Autodesk Inventor part; units mm, degrees
ref_plane "YZ Plane" through (0, 0, 0) normal (1, 0, 0) x (0, 1, 0)
ref_plane "XZ Plane" through (0, 0, 0) normal (0, 1, 0) x (-1, 0, 0)
ref_plane "XY Plane" through (0, 0, 0) normal (0, 0, 1) x (1, 0, 0)
sketch "Sketch1" plane through (0, 0, 0) normal (0, 1, 0) x (-1, 0, 0)
  line L0 (0, 0) -> (-25.4, 0)
  line L1 (-25.4, 0) -> (-25.4, 25.4)
  line L2 (-25.4, 25.4) -> (0, 25.4)
  line L3 (0, 25.4) -> (0, 0)
  line L4 (-1.5875, 23.8125) -> (-23.8125, 23.8125)
  line L5 (-23.8125, 23.8125) -> (-23.8125, 1.5875)
  line L6 (-23.8125, 1.5875) -> (-1.5875, 1.5875)
  line L7 (-1.5875, 1.5875) -> (-1.5875, 23.8125)
  dimension "d0" = 25.4
  dimension "d2" = 25.4
  dimension "d3" = 22.225
extrude "Extrusion1" add sketch "Sketch1" along normal blind 495.3
sketch "Sketch2" plane through (25.4, 0, 25.4) normal (1, 0, 0) x (0, 0, -1)
  line L0 (25.4, 0) -> (25.4, 495.3)
  line L1 (0, 495.3) -> (25.4, 495.3)
  line L2 (0, 495.3) -> (25.4, 469.9)
  point P0 (25.4, 25.4)
  dimension "d7" = 45
sketch "Sketch3" plane through (0, 0, 25.4) normal (-1, 0, 0) x (0, 0, 1)
  line L0 (0, 0) -> (0, 495.3)
  circle A0 centre (-6.35, 457.2) radius 3.3782
  circle A1 centre (-6.35, 431.8) radius 3.3782
  circle A2 centre (-6.35, 38.1) radius 3.3782
  circle A3 centre (-6.35, 63.5) radius 3.3782
  point P0 (-25.4, 0)
  dimension "d10" = 6.7564
  dimension "d11" = 6.7564
  dimension "d12" = 38.1
  dimension "d13" = 6.35
  dimension "d14" = 6.35
  dimension "d15" = 63.5
  dimension "d16" = 6.7564
  dimension "d17" = 6.7564
  dimension "d18" = 63.5
  dimension "d19" = 38.1
  dimension "d20" = 6.35
  dimension "d21" = 6.35
extrude "Extrusion3" cut sketch "Sketch3" against normal blind 25.4
ref_plane "Work Plane1" through (25.4, 25.4, 0) normal (0, 0, -1) x (-1, 0, 0)
sketch "Sketch4" plane through (25.4, 25.4, 0) normal (0, 0, -1) x (-1, 0, 0)
  circle A0 centre (12.6566, 207.0968) radius 3.3782
  circle A1 centre (12.6566, 168.9968) radius 3.3782
  point P0 (25.4, -25.4)
extrude "Extrusion4" cut sketch "Sketch4" against normal blind 25.4
sketch "Sketch5" plane through (25.4, 0, 25.4) normal (1, 0, 0) x (0, 0, -1)
  circle A0 centre (14.0716, 191.2218) radius 3.3782
  circle A1 centre (14.0716, 232.4968) radius 3.3782
  point P0 (25.4, 0)
extrude "Extrusion5" cut sketch "Sketch5" against normal blind 25.4
extrude "Extrusion6" cut sketch "Sketch2" against normal blind 25.4
sketch "Sketch8" plane through (0, 0, 0) normal (-1, 0, 0) x (0, 0, 1)
  circle A0 centre (12.7, 79.375) radius 3.3782
  circle A1 centre (12.7, 57.15) radius 3.3782
  circle A2 centre (12.7, 438.15) radius 3.3782
  circle A3 centre (12.7, 415.925) radius 3.3782
extrude "Extrusion9" cut sketch "Sketch8" against normal blind 25.4
sketch "Sketch9" plane through (25.4, 0, 0) normal (0, 0, -1) x (-1, 0, 0)
  circle A0 centre (12.7, 457.2) radius 3.3782
  circle A1 centre (12.7, 406.4) radius 3.3782
  circle A2 centre (12.7, 38.1) radius 3.3782
  circle A3 centre (12.7, 88.9) radius 3.3782
extrude "Extrusion10" cut sketch "Sketch9" against normal blind 25.4
sketch "Sketch10" plane through (0, 0, 0) normal (-1, 0, 0) x (0, 0, 1)
  circle A0 centre (19.05, 457.2) radius 3.3782
  circle A1 centre (19.05, 431.8) radius 3.3782
  circle A2 centre (19.05, 457.2) radius 3.3782
  circle A3 centre (19.05, 431.8) radius 3.3782
extrude "Extrusion11" add sketch "Sketch10" against normal blind 1.5875
sketch "Sketch11" plane through (25.4, 0, 25.4) normal (1, 0, 0) x (0, 0, -1)
  circle A0 centre (6.35, 431.8) radius 3.3782
  circle A1 centre (6.35, 457.2) radius 3.3782
  circle A2 centre (6.35, 457.2) radius 3.3782
  circle A3 centre (6.35, 431.8) radius 3.3782
extrude "Extrusion12" add sketch "Sketch11" against normal blind 1.5875
sketch "Sketch12" plane through (0, 0, 0) normal (-1, 0, 0) x (0, 0, 1)
  circle A0 centre (19.05, 38.1) radius 3.3782
  circle A1 centre (19.05, 63.5) radius 3.3782
  circle A2 centre (19.05, 63.5) radius 3.3782
  circle A3 centre (19.05, 38.1) radius 3.3782
extrude "Extrusion13" add sketch "Sketch12" against normal blind 1.5875
sketch "Sketch13" plane through (25.4, 0, 25.4) normal (1, 0, 0) x (0, 0, -1)
  circle A0 centre (6.35, 63.5) radius 3.3782
  circle A1 centre (6.35, 38.1) radius 3.3782
  circle A2 centre (6.35, 63.5) radius 3.3782
  circle A3 centre (6.35, 38.1) radius 3.3782
extrude "Extrusion14" add sketch "Sketch13" against normal blind 1.5875
properties part number "Square Tube" material "Aluminum 6061"
For this review, take the finished solid that the model builds, in its own axes (mm). A direction names the side the tool comes from. Round coordinates to 2 decimals unless told otherwise and drop trailing zeros. Write each loop counter-clockwise with the first axis right and the second up, starting at its lowest first coordinate (ties: lowest second). Pieces come first, ordered by that corner, then holes. Notation, with made-up numbers: (34, 88.25) - (53, 88.25) arc R27 cw to (53, 111.25) - close; hole circle Ø1 at (23.25, 24.5). An arc over 180 degrees is marked (long way). Answer as a JSON object with one key per item and string values.
1. To check wall thickness, follow line 1 along X through (y, z) = (32, 4.5); line 2 along X through (y, z) = (406.4, 24.85). State the ranges of each line that lie inside material, in increasing order.
Response values:
{"line 1": "x = 0 to 1.59, 23.81 to 25.4", "line 2": "x = 0 to 9.32, 16.08 to 25.4"}
2. Draft analysis for pull direction Z (two halves, no side actions). For faces 3 (the face through (13, 243, 23.812)), 4 (the face through (13, 244, 25.4)), 5 (the face through (24, 482.7, 12.8)), 6 (the face through (25.4, 244, 13)), state which applies: +Z half, -Z half, draft (parallel to the pull), parting line (faces both ways), or undercut.
Response values:
{"face 3": "undercut", "face 4": "+Z half", "face 5": "-Z half", "face 6": "draft"}
3. We need section B-B on y = 125.5. Give the boundary of the cut face in (x, z), then the cut area to 3 significant figures.
Response values:
{"outline": "(0, 0) - (25.4, 0) - (25.4, 25.4) - (0, 25.4) - close; hole (1.59, 1.59) - (23.81, 1.59) - (23.81, 23.81) - (1.59, 23.81) - close", "area": "151 mm2"}
4. We need section A-A on x = 20. Give the boundary of the cut face in (y, z), then the cut area to 3 significant figures.
Response values:
{"outline": "(0, 0) - (469.9, 0) - (471.49, 1.59) - (0, 1.59) - close; (0, 23.81) - (493.71, 23.81) - (495.3, 25.4) - (0, 25.4) - close", "area": "1,530 mm2"}
5. For pin 1 Ø6 at (x, z) = (12, 4.5) entering from +Y; pin 2 Ø12 at (x, z) = (16, 18.5) entering from +Y, all flat-tipped, find the tip position at first contact; note any pin that passes through.
Response values:
{"pin 1": "stops at y = 471.49", "pin 2": "stops at y = 494.4"}
6. Tool access review of faces 1 (the face through (24, 0, 13)), 2 (the face through (23.812, 243, 13)): name each direction out of +Z, -Z, +X, -X, +Y, -Y from which nothing blocks a thin tool from reaching the whole face with its end or side.
Response values:
{"face 1": "+Z, -Z, +X, -X, -Y", "face 2": "+Y, -Y"}
